The listing builds one solid part. Answer for the finished solid, in the listing's coordinates (mm). Give positions to 0.01 mm unless a question says otherwise; leave off trailing zeros. Loops run counter-clockwise (first coordinate to the right, second up) from the corner with the lowest first, then second, coordinate; pieces in that order, holes last. Notation, with made-up numbers: M 37,-7.5 L 49,-7.5 A29 ccw 49,12.5 Z; hole C 82,-33.75 d2. An arc over 180 degrees is marked long. One line per item, written item: value. Start each with the question number.
Q1. A cutting plane is placed at A-A, the plane z = -139. Determine the outline of the cut face in (x, y).
Q2. A cutting plane is placed at C-C, the plane z = -76. Determine the outline of the cut face in (x, y), and give its area (3 significant figures).
Q3. Flat-ended cylindrical pins translate along their axes: pin 1 (2.5 mm diameter, centred on x = 260, z = -90, fed in from +Y); pin 2 (1 mm diameter, centred on x = 140.5, y = 4, fed in from -Z). Find the tip coordinate at first contact, or state that the pin passes through.
Q4. Consider L1, parallel to X at y = 3.25, z = -20; L2, parallel to X at y = 1.2, z = -155; L3, parallel to X at y = 3.9, z = -131. Determine where each line is inside the solid, lowest interval first.
Q5. A cutting plane is placed at B-B, the plane y = 3.25. State how many separate pieces and enclosed holes the cut face has, and give its area (3 significant figures).
Autodesk Inventor part; units mm, degrees
ref_plane "YZ Plane" through (0, 0, 0) normal (1, 0, 0) x (0, 1, 0)
ref_plane "XZ Plane" through (0, 0, 0) normal (0, 1, 0) x (-1, 0, 0)
ref_plane "XY Plane" through (0, 0, 0) normal (0, 0, 1) x (1, 0, 0)
sketch "Sketch1" plane through (0, 0, 0) normal (0, 1, 0) x (-1, 0, 0)
  line L0 (0, 0) -> (-280, 0)
  line L1 (-280, 0) -> (-280, -190)
  line L2 (-280, -190) -> (0, -190)
  line L3 (5, -95) -> (-280, -95) construction
  line L4 (-140, 0) -> (-140, -190) construction
  line L5 (-57.5, 0) -> (-57.5, -190) construction
  line L6 (-203, 0) -> (-203, -190) construction
  line L7 (-20, -160) -> (-20, -130) construction
  line L8 (-20, -160) -> (-20, -130) construction
  line L9 (-17.75, -160) -> (-17.75, -130)
  line L10 (-22.25, -130) -> (-22.25, -160)
  arc A0 (-22.25, -160) -> (-17.75, -160) centre (-20, -160) ccw
  arc A1 (-17.75, -130) -> (-22.25, -130) centre (-20, -130) ccw
  line L11 (-95, -160) -> (-95, -130) construction
  line L12 (-95, -160) -> (-95, -130) construction
  line L13 (-97.25, -160) -> (-97.25, -130)
  line L14 (-92.75, -130) -> (-92.75, -160)
  arc A2 (-97.25, -160) -> (-92.75, -160) centre (-95, -160) ccw
  arc A3 (-92.75, -130) -> (-97.25, -130) centre (-95, -130) ccw
  line L15 (-160, -190) -> (-120, -190)
  line L16 (-120, -190) -> (-120, -185)
  line L17 (-120, -185) -> (-160, -185)
  line L18 (-160, -185) -> (-160, -190)
  line L19 (-260, -160) -> (-260, -130) construction
  line L20 (-260, -160) -> (-260, -130) construction
  line L21 (-262.25, -160) -> (-262.25, -130)
  line L22 (-257.75, -130) -> (-257.75, -160)
  arc A4 (-262.25, -160) -> (-257.75, -160) centre (-260, -160) ccw
  arc A5 (-257.75, -130) -> (-262.25, -130) centre (-260, -130) ccw
  line L23 (-187.25, -130) -> (-187.25, -160)
  line L24 (-185, -160) -> (-185, -130) construction
  line L25 (-182.75, -160) -> (-182.75, -130)
  arc A6 (-187.25, -160) -> (-182.75, -160) centre (-185, -160) ccw
  line L26 (-185, -160) -> (-185, -130) construction
  arc A7 (-182.75, -130) -> (-187.25, -130) centre (-185, -130) ccw
  line L27 (-140, -190) -> (-140, 0) construction
  line L28 (-20, -30) -> (-20, -60) construction
  line L29 (-20, -30) -> (-20, -60) construction
  line L30 (-17.75, -30) -> (-17.75, -60)
  line L31 (-22.25, -60) -> (-22.25, -30)
  arc A8 (-17.75, -30) -> (-22.25, -30) centre (-20, -30) ccw
  arc A9 (-22.25, -60) -> (-17.75, -60) centre (-20, -60) ccw
  line L32 (-92.75, -60) -> (-92.75, -30)
  line L33 (-95, -30) -> (-95, -60) construction
  line L34 (-97.25, -30) -> (-97.25, -60)
  arc A10 (-92.75, -30) -> (-97.25, -30) centre (-95, -30) ccw
  line L35 (-95, -30) -> (-95, -60) construction
  arc A11 (-97.25, -60) -> (-92.75, -60) centre (-95, -60) ccw
  line L36 (-160, 0) -> (-120, 0)
  line L37 (-120, 0) -> (-120, -5)
  line L38 (-120, -5) -> (-160, -5)
  line L39 (-160, -5) -> (-160, 0)
  arc A12 (-257.75, -30) -> (-262.25, -30) centre (-260, -30) ccw
  line L40 (-257.75, -60) -> (-257.75, -30)
  line L41 (-260, -30) -> (-260, -60) construction
  line L42 (-260, -30) -> (-260, -60) construction
  arc A13 (-262.25, -60) -> (-257.75, -60) centre (-260, -60) ccw
  line L43 (-262.25, -30) -> (-262.25, -60)
  line L44 (-187.25, -60) -> (-187.25, -30)
  line L45 (-185, -30) -> (-185, -60) construction
  line L46 (-185, -30) -> (-185, -60) construction
  arc A14 (-187.25, -60) -> (-182.75, -60) centre (-185, -60) ccw
  line L47 (-182.75, -30) -> (-182.75, -60)
  arc A15 (-182.75, -30) -> (-187.25, -30) centre (-185, -30) ccw
  line L48 (-280, -42.5) -> (-280, -92.5)
  line L49 (-280, -92.5) -> (-280, -145)
  line L50 (-280, -145) -> (-275, -145)
  line L51 (-275, -145) -> (-275, -45)
  line L52 (-275, -45) -> (-280, -45)
  line L53 (-280, -45) -> (-280, -42.5)
  line L54 (5, -45) -> (-5, -45)
  line L55 (-5, -45) -> (-5, -145)
  line L56 (-5, -145) -> (5, -145)
  line L57 (0, -190) -> (0, 0)
  point P0 (-20, -145)
  point P1 (-95, -145)
  point P2 (-260, -145)
  point P3 (-185, -145)
  point P4 (-20, -45)
  point P5 (-95, -45)
  point P6 (-260, -45)
  point P7 (-185, -45)
  point P8 (-95, -145)
  point P9 (-20, -145)
  point P10 (-280, -45)
  point P11 (-160, -190)
  point P12 (-120, -190)
  point P13 (-120, 0)
  point P14 (-160, 0)
  point P15 (-260, -145)
  point P16 (0, -45)
  point P17 (0, -145)
  dimension "d2" = 30
  dimension "d4" = 30
  dimension "d6" = 2.25
  dimension "d9" = 40
  dimension "d13" = 0
  dimension "d14" = 5
  dimension "d16" = 20
  dimension "d21" = 10
  dimension "d22" = 5
  dimension "d26" = 50
  dimension "d27" = 50
  dimension "d28" = 0
  dimension "d30" = 190
  dimension "d32" = 75
  dimension "d34" = 100
  dimension "d36" = 50
  dimension "d56" = 20
  dimension "d57" = 280
extrude "Extrusion1" add sketch "Sketch1" along normal blind 5 contours L57 L54 L55 L56 L2 L16 L17 L18 L1 L50 L51 L52 L0 L39 L38 L37
sketch "Sketch2" plane through (0, 5, 0) normal (0, 1, 0) x (1, 0, 0)
  line L0 (160, 185) -> (120, 185)
  line L1 (120, 185) -> (120, 190)
  line L2 (160, 5) -> (160, 0)
  line L3 (160, 0) -> (280, 0)
  line L4 (5, 145) -> (5, 45)
  point P0 (0, 0)
  point P1 (135, 20)
  point P2 (145, 20)
  point P3 (135, 170)
  point P4 (145, 170)
  point P5 (20, 90)
  point P6 (20, 100)
  dimension "d44" = 10
  dimension "d45" = 10
  dimension "d46" = 10
  dimension "d47" = 15
  dimension "d48" = 15
  dimension "d49" = 15
  dimension "d50" = 15
  dimension "d51" = 20
  dimension "d52" = 20
  dimension "d53" = 15
  dimension "d54" = 15
  dimension "d55" = 45
hole "Hole1" at (135, 5, -20) at (145, 5, -20) at (135, 5, -170) at (145, 5, -170) at (20, 5, -90) at (20, 5, -100) direction (0, -1, 0) diameter 4 end through all
sketch "Sketch3" plane through (0, 5, 0) normal (0, 1, 0) x (1, 0, 0)
  line L0 (275, 145) -> (280, 145)
  line L1 (275, 45) -> (275, 145)
  point P0 (0, 0)
  point P1 (260, 90)
  point P2 (260, 100)
  dimension "d65" = 45
  dimension "d66" = 10
  dimension "d67" = 15
  dimension "d68" = 15
hole "Hole2" at (260, 5, -90) at (260, 5, -100) direction (0, -1, 0) diameter 4 end through all
properties part number "base_2"
Answer block:
1. outline: M 5,0 L 17.75,0 L 17.75,5 L 5,5 Z; M 22.25,0 L 92.75,0 L 92.75,5 L 22.25,5 Z; M 97.25,0 L 182.75,0 L 182.75,5 L 97.25,5 Z; M 187.25,0 L 257.75,0 L 257.75,5 L 187.25,5 Z; M 262.25,0 L 275,0 L 275,5 L 262.25,5 Z
2. outline: M 5,0 L 275,0 L 275,5 L 5,5 Z
2. area: 1,350 mm^2
3. pin 1: through
3. pin 2: z = -185
4. L1: 0 to 133, 137 to 143, 147 to 280
4. L2: 0 to 17.75, 22.25 to 92.75, 97.25 to 182.75, 187.25 to 257.75, 262.25 to 280
4. L3: 5 to 17.75, 22.25 to 92.75, 97.25 to 182.75, 187.25 to 257.75, 262.25 to 275
5. separate pieces: 1
5. enclosed holes: 16
5. area: 50,500 mm^2
